from build123d import *

# Parameters (mm, degrees)
SKETCH_1_R      = 0.8
SKETCH_1_W      = 2
SKETCH_1_H      = 6
EXTRUDE_1_DEPTH = 3


with BuildPart() as part:
    # 草图1 → 凸台-拉伸1 (new body)
    with BuildSketch(Plane.XY):
        with BuildLine():
            Line((125, 20), (-125, 20))
            Line((-125, 20), (-125, -15))
            ThreePointArc((-125, -15), (-123.535533906, -18.535533906), (-120, -20))
            Line((-120, -20), (115, -20))
            ThreePointArc((115, -20), (122.071067812, -17.071067812), (125, -10))
            Line((125, -10), (125, 20))
        make_face()
        with BuildLine():
            Line((-117.577166779, -16.966576135), (-89.725823654, 9.134823104))
            ThreePointArc((-89.725823654, 9.134823104), (-88.308216305, 7.932037866), (-86.5, 7.5))
            Line((-86.5, 7.5), (-77.5, 7.5))
            ThreePointArc((-77.5, 7.5), (-75.2858442, 8.168706844), (-73.811998968, 9.951242954))
            Line((-73.811998968, 9.951242954), (-45.053835151, -17))
            Line((-45.053835151, -17), (-117, -17))
            ThreePointArc((-117, -17), (-117.28906688, -16.99163704), (-117.577166779, -16.966576135))
        make_face(mode=Mode.SUBTRACT)
        with BuildLine():
            Line((36.279498182, -17), (-36.279498182, -17))
            Line((-36.279498182, -17), (-3.41906176, 13.795763292))
            ThreePointArc((-3.41906176, 13.795763292), (0, 15.147473736), (3.41906176, 13.795763292))
            Line((3.41906176, 13.795763292), (36.279498182, -17))
        make_face(mode=Mode.SUBTRACT)
        with BuildLine():
            Line((112, -17), (45.053835151, -17))
            Line((45.053835151, -17), (77.914271574, 13.795763292))
            ThreePointArc((77.914271574, 13.795763292), (81.333333333, 15.147473736), (84.752395093, 13.795763292))
            Line((84.752395093, 13.795763292), (116.481383158, -15.93964233))
            ThreePointArc((116.481383158, -15.93964233), (114.302561258, -16.731300615), (112, -17))
        make_face(mode=Mode.SUBTRACT)
        with BuildLine():
            Line((-90.5, 12.520805239), (-120.487704725, -15.582724626))
            ThreePointArc((-120.487704725, -15.582724626), (-121.606436998, -13.944412041), (-122, -12))
            Line((-122, -12), (-122, 17))
            Line((-122, 17), (-90.5, 17))
            Line((-90.5, 17), (-90.5, 12.520805239))
        make_face(mode=Mode.SUBTRACT)
        with BuildLine():
            Line((-73.5, 17), (-4.387168485, 17))
            Line((-4.387168485, 17), (-37.247604907, -13.795763292))
            ThreePointArc((-37.247604907, -13.795763292), (-40.666666667, -15.147473736), (-44.085728426, -13.795763292))
            Line((-44.085728426, -13.795763292), (-73.5, 13.770363133))
            Line((-73.5, 13.770363133), (-73.5, 17))
        make_face(mode=Mode.SUBTRACT)
        with Locations((-85, 14.5)):
            Circle(SKETCH_1_R, mode=Mode.SUBTRACT)
        with Locations((-79, 14.5)):
            Circle(SKETCH_1_R, mode=Mode.SUBTRACT)
        with BuildLine():
            Line((4.387168485, 17), (76.946164849, 17))
            Line((76.946164849, 17), (44.085728426, -13.795763292))
            ThreePointArc((44.085728426, -13.795763292), (40.666666667, -15.147473736), (37.247604907, -13.795763292))
            Line((37.247604907, -13.795763292), (4.387168485, 17))
        make_face(mode=Mode.SUBTRACT)
        with BuildLine():
            ThreePointArc((122, -7), (121.212873995, -10.888824083), (118.975409451, -14.165449253))
            Line((118.975409451, -14.165449253), (99.406893969, 4.173545488))
            Line((99.406893969, 4.173545488), (102.055757879, 7))
            Line((102.055757879, 7), (122, 7))
            Line((122, 7), (122, -7))
        make_face(mode=Mode.SUBTRACT)
        with BuildLine():
            Line((100, 9.193584242), (97.217920236, 6.224982544))
            Line((97.217920236, 6.224982544), (85.720501818, 17))
            Line((85.720501818, 17), (98.687816207, 17))
            ThreePointArc((98.687816207, 17), (99.653283041, 15.859737408), (100, 14.406426589))
            Line((100, 14.406426589), (100, 9.193584242))
        make_face(mode=Mode.SUBTRACT)
        with Locations((104, 13)):
            Rectangle(SKETCH_1_W, SKETCH_1_H, mode=Mode.SUBTRACT)
        with Locations((118.5, 14.5)):
            Circle(SKETCH_1_R, mode=Mode.SUBTRACT)
        with Locations((112.5, 14.5)):
            Circle(SKETCH_1_R, mode=Mode.SUBTRACT)
    extrude(amount=EXTRUDE_1_DEPTH)


solid = part.part
Here's how the part is built. I have some questions about the finished solid (model axes, mm). A direction names the side the tool comes from. Give positions to 0.01 mm unless a question says otherwise; leave off trailing zeros. Answer as a JSON object with one key per item and string values. Group by question number.
Item 1: Will this pin go through, and if not, where does the flat tip stop? pin 1 (2.5 mm diameter, centred on x = 118.5, y = 14.5, fed in from +Z).
Item 2: Thinking about a two-plate mould opening in X: for faces 1 (the flat face through (9, 9, 3)), 2 (the flat face through (60.75, 1.82, 1.48)), 3 (the cylindrical face through (121.99, -17.15, 1.48)), which applies, pulls with the +X half, pulls with the -X half, needs draft (parallel to the pull), parting line crosses it, or undercut?
Item 3: On a 3-axis mill with a long thin cutter (end or side, diameter ignored), from which of +Z, -Z, +X, -X, +Y, -Y can I reach the whole of each face in a straight line? I mean faces 4 (the flat face through (9, 9, 0)), 5 (the flat face through (-103.85, -4.1, 1.48)). Say none if no direction works.
Item 4: I need wall thicknesses on L1, parallel to Y at x = -79, z = 0.9; L2, parallel to Y at x = 13, z = 0.15; L3, parallel to Y at x = -77, z = 2.75. Which ranges of each line are inside material? Lowest first, please.
Item 5: Imagine slicing it at A-A on z = 0.65. Give the number of separate pieces and of enclosed holes in the cut face, then the cut area to 3 significant figures.
Answer list:
{
 "1": {"pin 1": "stops at z = 3"},
 "2": {"face 1": "needs draft", "face 2": "undercut", "face 3": "pulls with the +X half"},
 "3": {"face 4": "-Z, +X, -X, +Y, -Y", "face 5": "+Z, -Z"},
 "4": {"L1": "y = -20 to -17, 7.5 to 13.7, 15.3 to 20", "L2": "y = -20 to -17, 4.82 to 8.93, 17 to 20", "L3": "y = -20 to -17, 7.53 to 20"},
 "5": {"separate pieces": "1", "enclosed holes": "13", "area": "2,920 mm2"}
}
